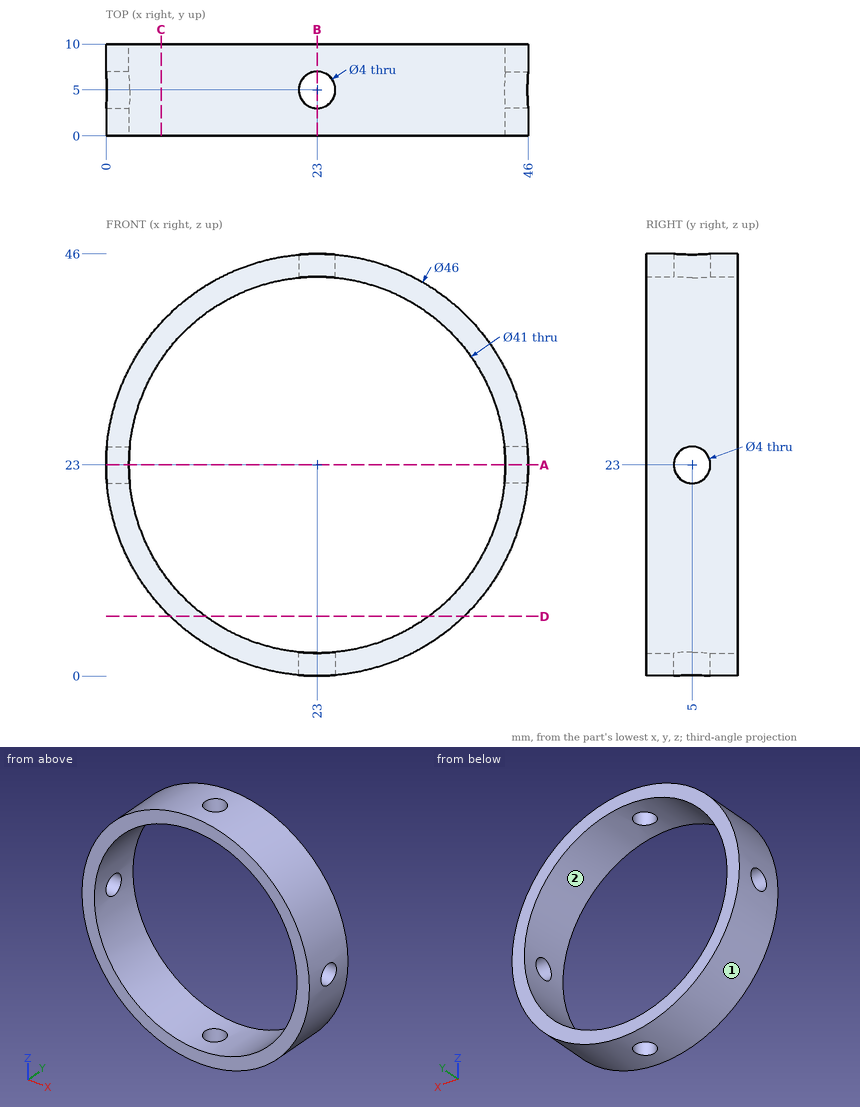
Drawing for the job (mm, zero at the part's lowest x, y, z). Give positions to 0.01 mm unless a question says otherwise; leave off trailing zeros. Loops run counter-clockwise (first coordinate to the right, second up) from the corner with the lowest first, then second, coordinate; pieces in that order, holes last.
Item 1: Slice it at D-D (z = 6.5). Write the cut outline in (x, y).
Check values:
outline: (6.98, 0) - (10.83, 0) - (10.83, 10) - (6.98, 10) - close; (35.17, 0) - (39.02, 0) - (39.02, 10) - (35.17, 10) - close
Item 2: Drill centre lines: line 1 along Y through (x, z) = (23, 44.3); line 2 along Z through (x, y) = (11, 9); line 3 along Z through (x, y) = (17, 8.25). Where is each one in solid material? Low to high.
Check values:
line 1: y = 0 to 3, 7 to 10
line 2: z = 3.38 to 6.38, 39.62 to 42.62
line 3: z = 0.8 to 3.4, 42.6 to 45.2
Item 3: Slice it at B-B (x = 23). Write the cut outline in (y, z), plus the area to 3 significant figures.
Check values:
outline: (0, 0) - (3, 0) - (3, 2.5) - (0, 2.5) - close; (0, 43.5) - (3, 43.5) - (3, 46) - (0, 46) - close; (7, 0) - (10, 0) - (10, 2.5) - (7, 2.5) - close; (7, 43.5) - (10, 43.5) - (10, 46) - (7, 46) - close
area: 30.0 mm2
Item 4: Drop flat-ended pins along their axis: P1, Ø5, axis at y = 7.5, z = 39, coming from the +X side; P2, Ø1, axis at y = 6.5, z = 13.5, coming from the +X side; P3, Ø3, axis at x = 28.5, y = 8, coming from the +Z side. Give the stop position or say it passes through.
Check values:
P1: stops at x = 41.62
P2: stops at x = 44.17
P3: stops at z = 45.65
Item 5: Slice it at A-A (z = 23). Write the cut outline in (x, y).
Check values:
outline: (0, 0) - (2.5, 0) - (2.5, 3) - (0, 3) - close; (0, 7) - (2.5, 7) - (2.5, 10) - (0, 10) - close; (43.5, 0) - (46, 0) - (46, 3) - (43.5, 3) - close; (43.5, 7) - (46, 7) - (46, 10) - (43.5, 10) - close
Item 6: Slice it at C-C (x = 6). Write the cut outline in (y, z).
Check values:
outline: (0, 7.51) - (10, 7.51) - (10, 11.54) - (0, 11.54) - close; (0, 34.46) - (10, 34.46) - (10, 38.49) - (0, 38.49) - close
Item 7: Mould opens along Z. For the marked faces 1 and 2 say: +Z half, -Z half, draft (parallel to the pull), parting line (faces both ways), or undercut.
Check values:
face 1: parting line
face 2: undercut
